Design review of the part built by this model. Coordinates are the model's own, in mm. A direction names the side the tool comes from. Give positions to 0.01 mm unless a question says otherwise; leave off trailing zeros. Write each loop counter-clockwise with the first axis right and the second up, starting at its lowest first coordinate (ties: lowest second). Pieces come first, ordered by that corner, then holes. Notation, with made-up numbers: (49, 27.5) -> (59, 27.5) arc R20 ccw to (59, 46.5) -> close; hole circle Ø4 at (89.25, -4.75). An arc over 180 degrees is marked (long way). Return JSON: item names as keys, results as strings. Group by question number.
from build123d import *

# Parameters (mm, degrees)
BOSS_EXTRUDE1_DEPTH      = 18
SKETCH4_R                = 3.975
BOSS_EXTRUDE2_DEPTH      = 10
BOSS_EXTRUDE2_DEPTH_BACK = 40


with BuildPart() as part:
    # Sketch1 → Boss-Extrude1 (new body)
    with BuildSketch(Plane.XY):
        with BuildLine():
            Line((0.700840098, 16.455896919), (0.810681557, 6.255896919))
            ThreePointArc((0.810681557, 6.255896919), (5.886159138, 8.587996721), (11.010681557, 6.365738378))
            Line((11.010681557, 6.365738378), (10.900840098, 16.565738378))
            Line((10.900840098, 16.565738378), (0.700840098, 16.455896919))
        make_face()
        with BuildLine():
            ThreePointArc((11.010681557, 6.365738378), (5.886159138, 8.587996721), (0.810681557, 6.255896919))
            Line((0.810681557, 6.255896919), (11.010681557, 6.365738378))
        make_face()
        with BuildLine():
            Line((11.010681557, 6.365738378), (0.810681557, 6.255896919))
            ThreePointArc((0.810681557, 6.255896919), (3.546395485, -4.672331118), (12.809920939, 1.738393871))
            ThreePointArc((12.809920939, 1.738393871), (12.344285051, 4.220811017), (11.010681557, 6.365738378))
        make_face()
    extrude(amount=BOSS_EXTRUDE1_DEPTH)

    # Sketch4 → Boss-Extrude2 (add, two sides)
    with BuildSketch(Plane(origin=(0, 0, 0), x_dir=(-1, 0, 0), z_dir=(0, 0, -1))) as boss_extrude2_sk:
        with Locations((-5.959920939, 1.738393871)):
            Circle(SKETCH4_R)
    extrude(amount=BOSS_EXTRUDE2_DEPTH)
    extrude(boss_extrude2_sk.sketch, amount=-BOSS_EXTRUDE2_DEPTH_BACK)


solid = part.part
Q1. Tool access review of faces 3 (the face through (2.288, 0.216, 28.846)), 4 (the face through (6, 2, 40)): name each direction out of +Z, -Z, +X, -X, +Y, -Y from which nothing blocks a thin tool from reaching the whole face with its end or side.
Q2. Insertion check: pin 1 (5 mm diameter, centred on x = 10.5, z = 18.5, fed in from -Y); pin 2 (2 mm diameter, centred on x = 1, y = -3, fed in from -Z); pin 3 (6 mm diameter, centred on x = 1.5, z = 30.5, fed in from +Y). Each pin has a flat end and moves straight along its axis. Give the tip position at first contact, or say it passes through.
Q3. Take a section at C-C, the plane z = 15.5. Give the boundary of the cut face in (x, y), plus the area to 3 significant figures.
Q4. Take a section at D-D, the plane z = 36. Give the boundary of the cut face in (x, y) (3 decimals), plus the area to 3 significant figures.
Q5. Take a section at A-A, the plane x = 2.75. Give the boundary of the cut face in (y, z).
Q6. Take a section at B-B, the plane y = 5. Give the boundary of the cut face in (x, z).
Q7. For L1, parallel to Z at x = 4, y = -2.75; L2, parallel to Y at x = 6, z = -8; L3, parallel to X at y = 15.75, z = 2, list the stretches that pass through material, from the lowest coordinate up. Write a range as from..to.
Q8. Mouldability with a two-part tool opening along Y and no side actions: class faces 1 (the face through (6, 2, -10)), 2 (the face through (2.288, 0.216, -4.93)) as +Y half, -Y half, draft (parallel to the pull), parting line (faces both ways), or undercut.
Final values:
{
 "1": {"face 3": "+Z", "face 4": "+Z, +X, -X, +Y, -Y"},
 "2": {"pin 1": "stops at y = -4.78", "pin 2": "stops at z = 0", "pin 3": "stops at y = 5.44"},
 "3": {"outline": "(0.7, 16.46) -> (0.81, 6.26) arc R6.85 ccw (long way) to (11.01, 6.37) -> (10.9, 16.57) -> close", "area": "235 mm²"},
 "4": {"outline": "circle Ø7.95 at (5.96, 1.738)", "area": "49.6 mm²"},
 "5": {"outline": "(-4.31, 0) -> (-0.61, 0) -> (-0.61, -10) -> (4.08, -10) -> (4.08, 0) -> (16.48, 0) -> (16.48, 18) -> (4.08, 18) -> (4.08, 40) -> (-0.61, 40) -> (-0.61, 18) -> (-4.31, 18) -> close"},
 "6": {"outline": "(-0.06, 0) -> (3.69, 0) -> (3.69, -10) -> (8.23, -10) -> (8.23, 0) -> (11.98, 0) -> (11.98, 18) -> (8.23, 18) -> (8.23, 40) -> (3.69, 40) -> (3.69, 18) -> (-0.06, 18) -> close"},
 "7": {"L1": "z = 0..18", "L2": "y = -2.24..5.71", "L3": "x = 0.71..10.91"},
 "8": {"face 1": "draft", "face 2": "parting line"}
}
